from build123d import *

# Parameters (mm, degrees)
SKETCH_1_R          = 5.03
SKETCH_1_R_2        = 1.25
SKETCH_1_R_3        = 1.5
EXTRUDE_1_DEPTH     = 3
SKETCH_2_R          = 2
CUT_EXTRUDE_1_DEPTH = 4


with BuildPart() as part:
    # 草图1 → 凸台-拉伸1 (new body)
    with BuildSketch(Plane.XY):
        with BuildLine():
            Line((-15.488984032, 1), (-9.488984032, 1))
            ThreePointArc((-9.488984032, 1), (-4.998995168, 4.6), (-0.509006304, 1))
            Line((-0.509006304, 1), (5.001004832, 1))
            Line((5.001004832, 1), (39.254812875, 1))
            Line((39.254812875, 1), (39.254812875, 3.326018382))
            Line((39.254812875, 3.326018382), (5.001004832, 11.501004832))
            Line((5.001004832, 11.501004832), (-38.998995168, 22.002009663))
            ThreePointArc((-38.998995168, 22.002009663), (-61.001004832, 0), (-38.998995168, -22.002009663))
            Line((-38.998995168, -22.002009663), (5.001004832, -11.501004832))
            Line((5.001004832, -11.501004832), (5.001004832, -1))
            Line((5.001004832, -1), (-0.509006304, -1))
            ThreePointArc((-0.509006304, -1), (-4.998995168, -4.6), (-9.488984032, -1))
            Line((-9.488984032, -1), (-15.488984032, -1))
            Line((-15.488984032, -1), (-15.488984032, 1))
        make_face()
        with Locations((-38.998995168, 0)):
            Circle(SKETCH_1_R, mode=Mode.SUBTRACT)
        with Locations((-38.998995168, -11.5)):
            Circle(SKETCH_1_R_2, mode=Mode.SUBTRACT)
        with Locations((-12.498995168, -10)):
            Circle(SKETCH_1_R_3, mode=Mode.SUBTRACT)
        with Locations((-22.498995168, 0)):
            Circle(SKETCH_1_R_3, mode=Mode.SUBTRACT)
        with Locations((-48.958287312, -5.75)):
            Circle(SKETCH_1_R_2, mode=Mode.SUBTRACT)
        with Locations(Location((-12.498995168, 10, 0), (0, 0, 180))):
            Circle(SKETCH_1_R_3, mode=Mode.SUBTRACT)
        with Locations((-48.958287312, 5.75)):
            Circle(SKETCH_1_R_2, mode=Mode.SUBTRACT)
        with Locations((-38.998995168, 11.5)):
            Circle(SKETCH_1_R_2, mode=Mode.SUBTRACT)
        with Locations((-29.039703025, 5.75)):
            Circle(SKETCH_1_R_2, mode=Mode.SUBTRACT)
        with Locations((-29.039703025, -5.75)):
            Circle(SKETCH_1_R_2, mode=Mode.SUBTRACT)
    extrude(amount=EXTRUDE_1_DEPTH)

    # 草图2 → 切除-拉伸1 (cut)
    with BuildSketch(Plane(origin=(0, 0, 0), x_dir=(-1, 0, 0), z_dir=(0, 0, -1))):
        with Locations((0, 12.694540648)):
            Circle(SKETCH_2_R)
        with Locations((0, -12.694540648)):
            Circle(SKETCH_2_R)
    extrude(amount=-CUT_EXTRUDE_1_DEPTH, mode=Mode.SUBTRACT)


solid = part.part
Check sheet for the modelled part. Datum: model origin and axes. Units: mm. A direction names the side the tool comes from. Round coordinates to 2 decimals unless told otherwise and drop trailing zeros. Loops run counter-clockwise (first coordinate to the right, second up) from the corner with the lowest first, then second, coordinate; pieces in that order, holes last. Notation, with made-up numbers: (64, -28.5) -> (110, -28.5) arc R19 ccw to (110, 2.5) -> close; hole circle Ø7 at (56, -32.5). An arc over 180 degrees is marked (long way). Put each result on its own line as item: value. Start each with the question number.
1. Access from +Z, -Z, +X, -X, +Y, -Y to the whole of each face (thin tool, end or side, straight path). Record for faces 4 (the face through (39.255, 2, 1)), 5 (the face through (-5.1, 4.6, 1.5)), 6 (the face through (-15.489, 0, 1)).
2. Scan lines: probe 1 along Y at (x, z) = (-39, 1.85); probe 2 along Y at (x, z) = (-38.5, 2.6); probe 3 along X at (y, z) = (-2, 1.15). Record each from-to range of solid material in increasing order.
3. Draft check along Y on faces 1 (the face through (-20.73, -17.64, 1.48)), 2 (the face through (2, -1, 1)), 3 (the face through (-61, 0, 1)). Enter one of: +Y half, -Y half, draft (parallel to the pull), parting line (faces both ways), or undercut.
4. Section check C-C (x = -7). Enter the section's corners in (y, z).
5. Section check B-B (z = 1.95). Give the number of separate pieces and of enclosed holes in the cut face, plus the area to 3 significant figures.
6. Section check A-A (y = 0). Enter the section's corners in (x, z), plus the area to 3 significant figures.
7. Section check D-D (x = 20). Enter the section's corners in (y, z).
8. Gauge pin test, flat ends, axial feed: pin 1 (1.8 mm diameter, centred on x = -12.5, y = 10, fed in from -Z); pin 2 (4 mm diameter, centred on x = -29.04, y = -5.75, fed in from +Z); pin 3 (1 mm diameter, centred on x = 25, z = 1, fed in from -Y). Record the tip position at first contact, or that the pin passes through.
Findings:
1. face 4: +Z, -Z, +X, +Y, -Y
1. face 5: +Z, -Z
1. face 6: +Z, -Z, +X
2. probe 1: y = -22 to -12.75, -10.25 to -5.03, 5.03 to 10.25, 12.75 to 22
2. probe 2: y = -21.88 to -12.65, -10.35 to -5.01, 5.01 to 10.35, 12.65 to 21.88
2. probe 3: x = -60.91 to -43.61, -34.38 to -9.14, -0.86 to 5
3. face 1: -Y half
3. face 2: undercut
3. face 3: parting line
4. outline: (-14.37, 0) -> (-4.14, 0) -> (-4.14, 3) -> (-14.37, 3) -> close; (4.14, 0) -> (14.37, 0) -> (14.37, 3) -> (4.14, 3) -> close
5. separate pieces: 1
5. enclosed holes: 10
5. area: 2,220 mm^2
6. outline: (-61, 0) -> (-44.03, 0) -> (-44.03, 3) -> (-61, 3) -> close; (-33.97, 0) -> (-24, 0) -> (-24, 3) -> (-33.97, 3) -> close; (-21, 0) -> (-15.49, 0) -> (-15.49, 3) -> (-21, 3) -> close
6. area: 97.4 mm^2
7. outline: (1, 0) -> (7.92, 0) -> (7.92, 3) -> (1, 3) -> close
8. pin 1: passes through
8. pin 2: stops at z = 3
8. pin 3: stops at y = 1
